Work out the finished part from the listing and answer in its coordinate system (mm). A direction names the side the tool comes from. Coordinates: 2 decimals unless noted, no trailing zeros. Order: outer loops, then holes, each group sorted by start corner. A loop starts at its lowest first (then second) coordinate and runs counter-clockwise, first axis right, second up. Notation, with made-up numbers: M -26,18 L 18,18 A29 cw 18,52 Z; hole C 85.25,-37.5 d8. An arc over 180 degrees is marked long. Answer in a Markdown table with one row per item. Add a question column.
Item 1: The mould has two halves that part along X. Classify faces 1 (the face through (23.786, -0.986, -31.494)), 2 (the face through (150, -39, -26)), 3 (the face through (74, -2, -30)), 4 (the face through (74, -39, -50)): released by +X, released by -X, zero draft, split by the parting line, or undercut.
Item 2: The part is cut by section B-B (z = -25). Write down the section's boundary in (x, y), then the cut area to 3 significant figures.
Item 3: Which of the six approach directions +Z, -Z, +X, -X, +Y, -Y give full straight-line access (tool end or side, diameter ignored) to faces 5 (the face through (66.095, -0.986, -25.867)), 6 (the face through (74, 0, -26.3)), 7 (the face through (74, -78, -25))?
Item 4: Flat-ended cylindrical pins translate along their axes: pin 1 Ø21.5 at (x, z) = (94.75, -25) entering from +Y; pin 2 Ø1.5 at (x, y) = (52, -12.5) entering from +Z; pin 3 Ø8 at (x, z) = (48, -25) entering from +Y. Find the tip coordinate at first contact, or state that the pin passes through.
Item 5: The part is cut by section D-D (x = 70). Write down the section's boundary in (y, z).
Item 6: Consider line 1 (X direction, y = -1.45, z = -25); line 2 (Y direction, x = 131, z = -37.5); line 3 (X direction, y = -48, z = -6). Determine where each line is inside the solid, lowest interval first. Write a range as from..to.
Item 7: The part is cut by section C-C (z = -14). Write down the section's boundary in (x, y).
Item 8: The part is cut by section A-A (x = 94.75). Write down the section's boundary in (y, z).
from build123d import *

# Parameters (mm, degrees)
SKETCH1_W          = 150
SKETCH1_H          = 50
EXTRUDE5_DEPTH     = 80
SHELL1_T           = 2
EXTRUDE6_REACH     = 82
SKETCH8_R          = 6.5
SKETCH8_R_2        = 6.75
SKETCH8_R_3        = 4
SKETCH8_R_4        = 6
SKETCH12_W         = 2
SKETCH12_H         = 80
CUT_EXTRUDE1_DEPTH = 200


with BuildPart() as part:
    # Sketch1 → Extrude5 (new body)
    with BuildSketch(Plane(origin=(0, 0, 0), x_dir=(1, 0, 0), z_dir=(0, 1, 0))):
        with Locations((75, 25)):
            Rectangle(SKETCH1_W, SKETCH1_H)
    extrude(amount=-EXTRUDE5_DEPTH)

    # Shell1 (no face opened: a closed hollow body)
    add(offset(amount=-SHELL1_T, mode=Mode.PRIVATE), mode=Mode.SUBTRACT)

    # Sketch8 → Extrude6 (cut, up to next)
    with BuildSketch(Plane(origin=(0, 0, 0), x_dir=(1, 0, 0), z_dir=(0, 1, 0)), mode=Mode.PRIVATE) as extrude6_sk1:
        with Locations(Location((23.5, 25, 0), (0, 0, 270))):  # turned: the seam where the file's is
            Circle(SKETCH8_R)
    extrude6_tool1 = extrude(extrude6_sk1.sketch, amount=-EXTRUDE6_REACH, mode=Mode.PRIVATE) & part.part
    add(extrude6_tool1.solids().sort_by_distance((23.5, 0, -25))[0], mode=Mode.SUBTRACT)
    # Sketch8 → Extrude6 (cut, up to next)
    with BuildSketch(Plane(origin=(0, 0, 0), x_dir=(1, 0, 0), z_dir=(0, 1, 0)), mode=Mode.PRIVATE) as extrude6_sk2:
        with Locations(Location((48, 25, 0), (0, 0, 270))):  # turned: the seam where the file's is
            Circle(SKETCH8_R_2)
    extrude6_tool2 = extrude(extrude6_sk2.sketch, amount=-EXTRUDE6_REACH, mode=Mode.PRIVATE) & part.part
    add(extrude6_tool2.solids().sort_by_distance((48, 0, -25))[0], mode=Mode.SUBTRACT)
    # Sketch8 → Extrude6 (cut, up to next)
    with BuildSketch(Plane(origin=(0, 0, 0), x_dir=(1, 0, 0), z_dir=(0, 1, 0)), mode=Mode.PRIVATE) as extrude6_sk3:
        with Locations(Location((70, 25, 0), (0, 0, 270))):  # turned: the seam where the file's is
            Circle(SKETCH8_R_3)
    extrude6_tool3 = extrude(extrude6_sk3.sketch, amount=-EXTRUDE6_REACH, mode=Mode.PRIVATE) & part.part
    add(extrude6_tool3.solids().sort_by_distance((70, 0, -25))[0], mode=Mode.SUBTRACT)
    # Sketch8 → Extrude6 (cut, up to next)
    with BuildSketch(Plane(origin=(0, 0, 0), x_dir=(1, 0, 0), z_dir=(0, 1, 0)), mode=Mode.PRIVATE) as extrude6_sk4:
        with Locations(Location((94.75, 25, 0), (0, 0, 270))):  # turned: the seam where the file's is
            Circle(SKETCH8_R_2)
    extrude6_tool4 = extrude(extrude6_sk4.sketch, amount=-EXTRUDE6_REACH, mode=Mode.PRIVATE) & part.part
    add(extrude6_tool4.solids().sort_by_distance((94.75, 0, -25))[0], mode=Mode.SUBTRACT)
    # Sketch8 → Extrude6 (cut, up to next)
    with BuildSketch(Plane(origin=(0, 0, 0), x_dir=(1, 0, 0), z_dir=(0, 1, 0)), mode=Mode.PRIVATE) as extrude6_sk5:
        with Locations(Location((124, 25, 0), (0, 0, 270))):  # turned: the seam where the file's is
            Circle(SKETCH8_R_4)
    extrude6_tool5 = extrude(extrude6_sk5.sketch, amount=-EXTRUDE6_REACH, mode=Mode.PRIVATE) & part.part
    add(extrude6_tool5.solids().sort_by_distance((124, 0, -25))[0], mode=Mode.SUBTRACT)

    # Sketch12 → Cut-Extrude1 (cut)
    with BuildSketch(Plane.ZY):
        with Locations((-1, -40)):
            Rectangle(SKETCH12_W, SKETCH12_H)
    extrude(amount=-CUT_EXTRUDE1_DEPTH, mode=Mode.SUBTRACT)


solid = part.part
Reply:
| question | item | result |
|---|---|---|
| 1 | face 1 | undercut |
| 1 | face 2 | released by +X |
| 1 | face 3 | undercut |
| 1 | face 4 | zero draft |
| 2 | outline | M 0,-80 L 150,-80 L 150,0 L 130,0 L 130,-2 L 148,-2 L 148,-78 L 2,-78 L 2,-2 L 17,-2 L 17,0 L 0,0 Z; M 30,-2 L 41.25,-2 L 41.25,0 L 30,0 Z; M 54.75,-2 L 66,-2 L 66,0 L 54.75,0 Z; M 74,-2 L 88,-2 L 88,0 L 74,0 Z; M 101.5,-2 L 118,-2 L 118,0 L 101.5,0 Z |
| 2 | area | 784 mm2 |
| 3 | face 5 | +Y |
| 3 | face 6 | +Z, -Z, +X, -X, +Y |
| 3 | face 7 | +Z |
| 4 | pin 1 | stops at y = 0 |
| 4 | pin 2 | stops at z = -48 |
| 4 | pin 3 | stops at y = -78 |
| 5 | outline | M -80,-50 L 0,-50 L 0,-29 L -2,-29 L -2,-48 L -78,-48 L -78,-2 L -80,-2 Z; M -2,-21 L 0,-21 L 0,-2 L -2,-2 Z |
| 6 | line 1 | x = 0..17, 30..41.25, 54.75..66, 74..88, 101.5..118, 130..150 |
| 6 | line 2 | y = -80..-78, -2..0 |
| 6 | line 3 | x = 0..2, 148..150 |
| 7 | outline | M 0,-80 L 150,-80 L 150,0 L 0,0 Z; hole M 2,-78 L 148,-78 L 148,-2 L 2,-2 Z |
| 8 | outline | M -80,-50 L 0,-50 L 0,-31.75 L -2,-31.75 L -2,-48 L -78,-48 L -78,-2 L -80,-2 Z; M -2,-18.25 L 0,-18.25 L 0,-2 L -2,-2 Z |
